The drawing under review shows one solid part. Ordinate dimensions are in mm from its lowest x, y, z. A direction names the side the tool comes from. Round coordinates to 2 decimals unless told otherwise and drop trailing zeros. Write item = value, one per line. Start each with the question number.
Item 1: For pin 1 Ø4 at (x, y) = (4.6, 18.42) entering from +Z; pin 2 Ø5 at (y, z) = (21, 4) entering from -X; pin 3 Ø4 at (y, z) = (28.5, 4.5) entering from +X, all flat-tipped, find the tip position at first contact; note any pin that passes through.
Item 2: To check wall thickness, follow line 1 along Y through (x, z) = (4, 2.25); line 2 along Y through (x, z) = (4.75, 5.75); line 3 along X through (y, z) = (8, 4.75) (1 decimal). State the ranges of each line that lie inside material, in increasing order.
Item 3: The part is to be moulded in two halves that separate along Y. For the marked faces 1, 2 and 3, say which applies: +Y half, -Y half, draft (parallel to the pull), parting line (faces both ways), or undercut.
Item 4: Tool access review of the marked faces 4 and 5: name each direction out of +Z, -Z, +X, -X, +Y, -Y from which nothing blocks a thin tool from reaching the whole face with its end or side.
Item 5: Take a section at B-B, the plane z = 4.25. Give the number of separate pieces and of enclosed holes in the cut face.
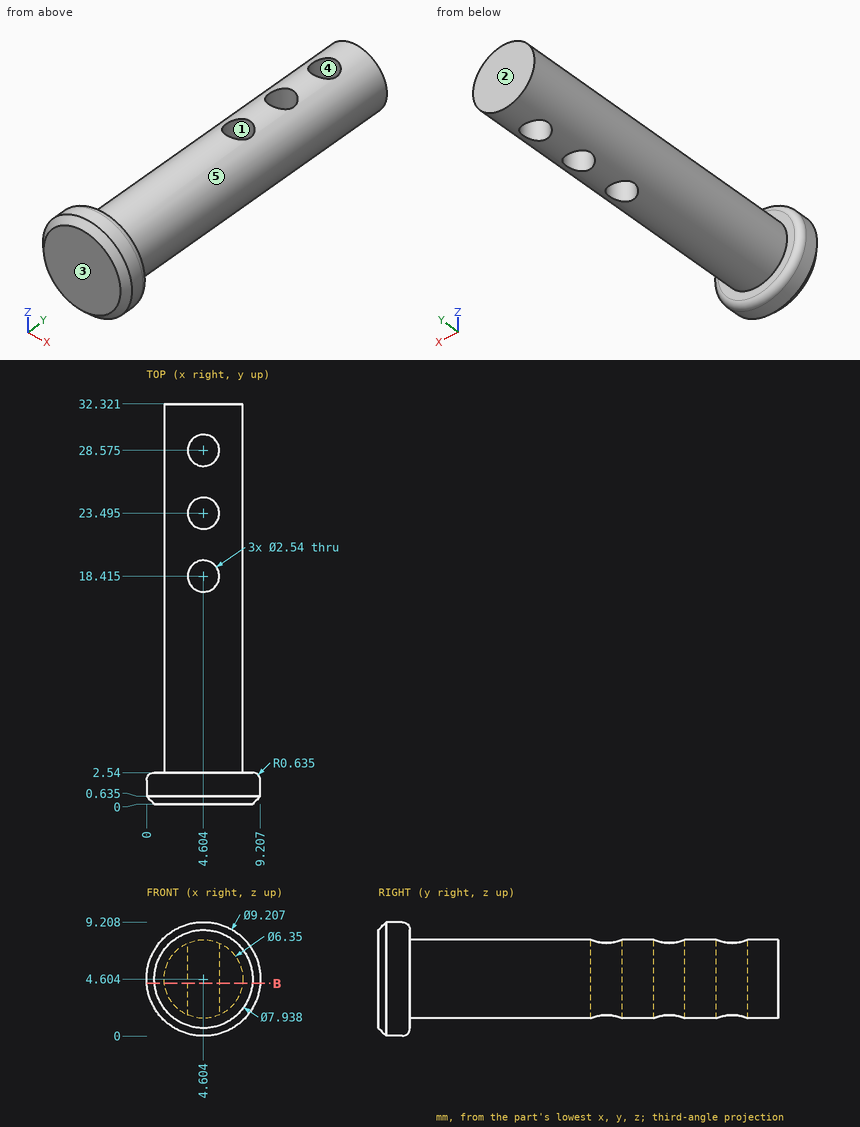
Response values:
q1.pin_1 = 7.78
q1.pin_2 = 1.43
q1.pin_3 = 7.78
q2.line_1 = 0 to 17.3, 19.53 to 22.38, 24.61 to 27.46, 29.69 to 32.32
q2.line_2 = 0 to 17.15, 19.68 to 22.23, 24.76 to 27.31, 29.84 to 32.32
q2.line_3 = 1.4 to 7.8
q3.face_1 = undercut
q3.face_2 = +Y half
q3.face_3 = -Y half
q4.face_4 = +Z, -Z
q4.face_5 = +Y
q5.separate_pieces = 1
q5.enclosed_holes = 3
